Here's the drawing with two shaded views (mm, measured from the low corner). I have some questions. Coordinates: 2 decimals unless noted, no trailing zeros. Write each loop counter-clockwise with the first axis right and the second up, starting at its lowest first coordinate (ties: lowest second). Pieces come first, ordered by that corner, then holes.
Item 1: I want a section at C-C on z = 3.5. Please give me the cut outline in (x, y), then the cut area to 3 significant figures.
Item 2: For P1, Ø2, axis at y = 6.5, z = 8.5, coming from the -X side; P2, Ø3.5, axis at x = 4, y = 4, coming from the -Z side; P3, Ø3, axis at y = 6.5, z = 10.5, coming from the +X side; P4, Ø4, axis at y = 3.5, z = 4.5, coming from the +X side, each with a flat end and sliding along its axis, tell me the tip position at first contact or that it passes through.
Item 3: I want a section at A-A on x = 4. Please give me the cut outline in (y, z), then the cut area to 3 significant figures.
Item 4: If I drill on probe 1 along Y at (x, z) = (4, 8); probe 2 along X at (y, z) = (5.25, 4); probe 3 along X at (y, z) = (2.5, 1), over which ranges is the centre line in solid material (lowest first)?
Item 5: Thinking about a two-plate mould opening in Y: for the marked faces 1, 2 and 3, which applies, +Y half, -Y half, draft (parallel to the pull), parting line (faces both ways), or undercut?
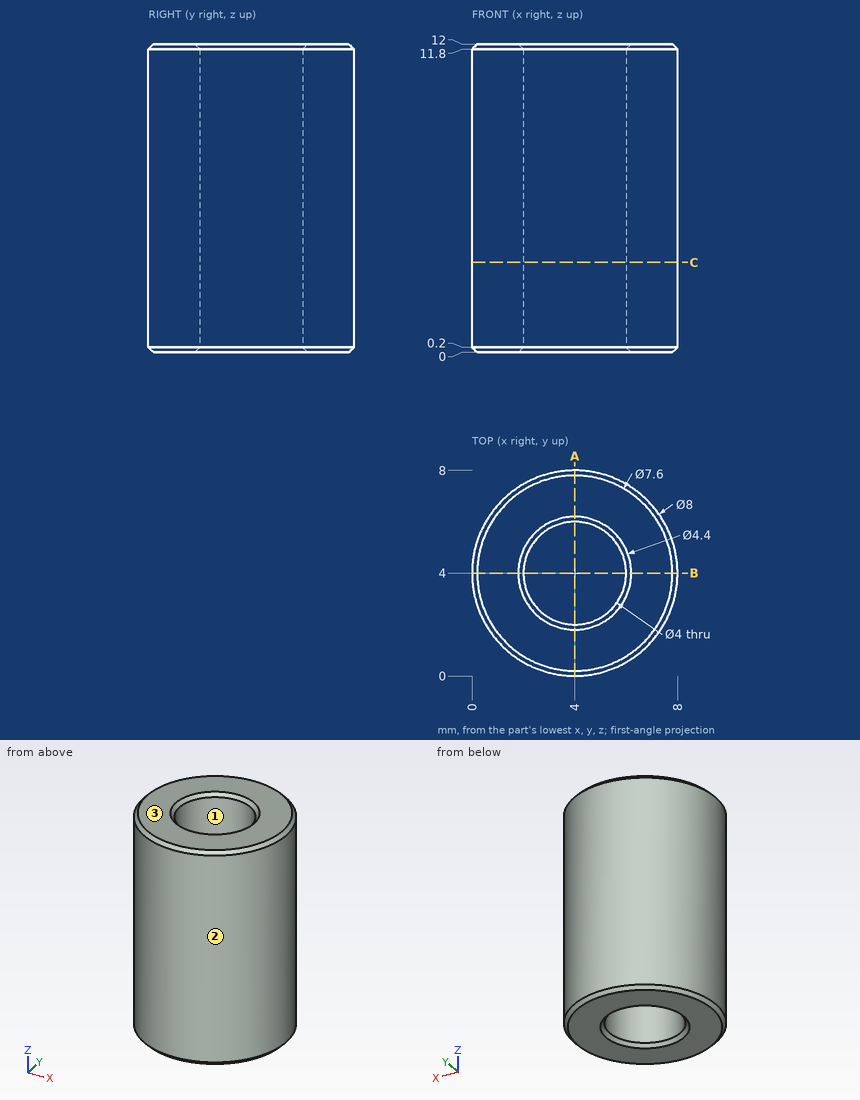
Response values:
1. outline: circle Ø8 at (4, 4); hole circle Ø4 at (4, 4)
1. area: 37.7 mm2
2. P1: stops at x = 0.29
2. P2: passes through
2. P3: stops at x = 7.87
2. P4: stops at x = 8
3. outline: (0, 0.2) - (0.2, 0) - (1.8, 0) - (2, 0.2) - (2, 11.8) - (1.8, 12) - (0.2, 12) - (0, 11.8) - close; (6, 0.2) - (6.2, 0) - (7.8, 0) - (8, 0.2) - (8, 11.8) - (7.8, 12) - (6.2, 12) - (6, 11.8) - close
3. area: 47.8 mm2
4. probe 1: y = 0 to 2, 6 to 8
4. probe 2: x = 0.2 to 2.44, 5.56 to 7.8
4. probe 3: x = 0.29 to 2.68, 5.32 to 7.71
5. face 1: undercut
5. face 2: parting line
5. face 3: draft
